Check sheet for the modelled part. Datum: model origin and axes. Units: mm. Round coordinates to 2 decimals unless told otherwise and drop trailing zeros. Order: outer loops, then holes, each group sorted by start corner. A loop starts at its lowest first (then second) coordinate and runs counter-clockwise, first axis right, second up.
Q1. Cross-section at C-C on x = 4.5. Record the cut outline in (y, z), then the cut area to 3 significant figures.
Q2. Depth check by flat-ended pin: P1, Ø1.5, axis at x = -1.5, y = 42.5, coming from the -Z side. Enter the tip coordinate at first touch or a pass-through.
Q3. Scan lines: probe 1 along Y at (x, z) = (-2.25, 13.25); probe 2 along Y at (x, z) = (3, 12.75); probe 3 along Z at (x, y) = (5.75, -85). Record each from-to range of solid material in increasing order.
Q4. Cross-section at A-A on z = 12.5. Record the cut outline in (x, y), then the cut area to 3 significant figures.
Q5. Cross-section at D-D on y = 175. Record the cut outline in (x, z).
Q6. Cross-section at B-B on y = -85. Record the cut outline in (x, z).
Q7. Mould release check, pull along Z, two halves, no side actions. Record for faces 1 (the cylindrical face through (-0.175, -20.504, 12.698)), 2 (the flat face through (0, 264, 0)), 3 (the flat face through (0, 264, 25)): +Z half, -Z half, draft (parallel to the pull), parting line (faces both ways), or undercut.
from build123d import *

# Parameters (mm, degrees)
F0_W          = 350
F0_H          = 25
F1_DEPTH      = 12.5
F1_DEPTH_BACK = 12.5
F3_DEPTH      = 25
F5_DEPTH      = 100
F7_D          = 9


# Not quite as in the source:
# - a pattern or mirror of a feature is missing from the dataset's text; its kind, count and spacing are read off the source's solid


with BuildPart() as f1:
    # F0 (on Right) → F1 (new body, two sides)
    with BuildSketch(Plane.YZ) as f1_sk:
        with Locations((175, 12.5)):
            Rectangle(F0_W, F0_H)
    extrude(amount=F1_DEPTH)
    extrude(f1_sk.sketch, amount=-F1_DEPTH_BACK)

    # F2 (on face) → F3 (cut)
    with BuildSketch(Plane.YZ.offset(12.5)):
        with BuildLine():
            ThreePointArc((169, 25), (175, 19), (181, 25))
            Line((181, 25), (169, 25))
        make_face()
    f3 = extrude(amount=-F3_DEPTH, mode=Mode.SUBTRACT)

    # F3_copies: F3 across plane
    add(f3.mirror(Plane(origin=(0, 0, 12.5), x_dir=(-1, 0, 0), z_dir=(0, 0, -1))), mode=Mode.SUBTRACT)

    # F5 (add): a face of the model
    f5_faces = [f1.faces().sort_by_distance(p)[0] for p in [
        (0, 0, 12.5),
    ]]
    extrude(f5_faces, amount=F5_DEPTH)

    # F7 (through all)
    with Locations(Plane.YZ.offset(12.5)):
        with Locations((-85, 12.5), (-55, 12.5), (-25, 12.5)):
            Hole(F7_D / 2)


solid = f1.part
Results found:
1. outline: (-100, 0) - (169, 0) arc R6 cw to (181, 0) - (350, 0) - (350, 25) - (181, 25) arc R6 cw to (169, 25) - (-100, 25) - close; hole circle Ø9 at (-85, 12.5); hole circle Ø9 at (-55, 12.5); hole circle Ø9 at (-25, 12.5)
1. area: 10,900 mm2
2. P1: stops at z = 0
3. probe 1: y = -100 to -89.44, -80.56 to -59.44, -50.56 to -29.44, -20.56 to 350
3. probe 2: y = -100 to -89.49, -80.51 to -59.49, -50.51 to -29.49, -20.51 to 350
3. probe 3: z = 0 to 8, 17 to 25
4. outline: (-12.5, -100) - (12.5, -100) - (12.5, -89.5) - (-12.5, -89.5) - close; (-12.5, -80.5) - (12.5, -80.5) - (12.5, -59.5) - (-12.5, -59.5) - close; (-12.5, -50.5) - (12.5, -50.5) - (12.5, -29.5) - (-12.5, -29.5) - close; (-12.5, -20.5) - (12.5, -20.5) - (12.5, 350) - (-12.5, 350) - close
4. area: 10,600 mm2
5. outline: (-12.5, 6) - (12.5, 6) - (12.5, 19) - (-12.5, 19) - close
6. outline: (-12.5, 0) - (12.5, 0) - (12.5, 8) - (-12.5, 8) - close; (-12.5, 17) - (12.5, 17) - (12.5, 25) - (-12.5, 25) - close
7. face 1: undercut
7. face 2: -Z half
7. face 3: +Z half
